Input: part model. Units: mm. Frame: model coordinates. Coordinates: 2 decimals unless noted, no trailing zeros. Write each loop counter-clockwise with the first axis right and the second up, starting at its lowest first coordinate (ties: lowest second). Pieces come first, ordered by that corner, then holes.
1) Section query C-C (z = 36). Output: boundary loops of the cut face in (x, y).
2) Line query: L1, parallel to Z at x = -1, y = 0.75; L2, parallel to X at y = 0.9, z = 45.5; L3, parallel to X at y = 0.7, z = -29.5. Output: solid intervals per line, ascending.
3) Section query B-B (x = -35). Output: boundary loops of the cut face in (y, z), then the cut area to 3 significant figures.
4) Section query A-A (y = 0.45). Output: boundary loops of the cut face in (x, z), then the cut area to 3 significant figures.
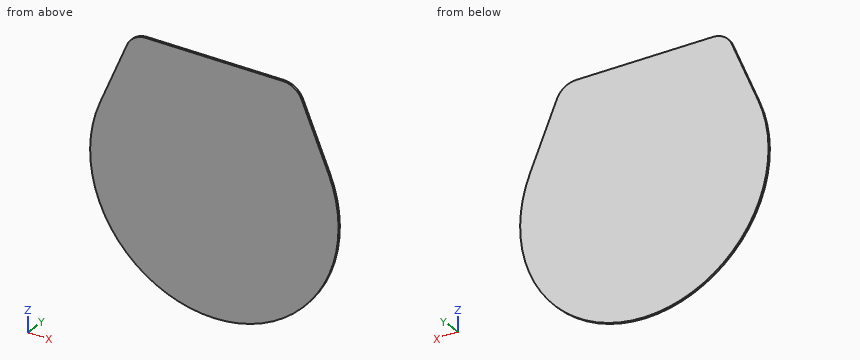
from build123d import *

# Parameters (mm, degrees)
SKETCH1_R           = 60.5
BOSS_EXTRUDE1_DEPTH = 1
BOSS_EXTRUDE2_START = -1
BOSS_EXTRUDE2_DEPTH = 1
FILLET1_R           = 10


with BuildPart() as part:
    # Sketch1 → Boss-Extrude1 (new body)
    with BuildSketch(Plane(origin=(0, 0, 0), x_dir=(1, 0, 0), z_dir=(0, 1, 0))):
        with Locations(Location((0, 0, 0), (0, 0, 270))):
            Circle(SKETCH1_R)
    extrude(amount=BOSS_EXTRUDE1_DEPTH)

    # Sketch7 → Boss-Extrude2 (add)
    with BuildSketch(Plane(origin=(0, 1, 0), x_dir=(1, 0, 0), z_dir=(0, 1, 0)).offset(BOSS_EXTRUDE2_START)):
        with BuildLine():
            Line((-55.577310907, -23.904236284), (-40, -60.5))
            Line((-40, -60.5), (2.22e-07, -60.5))
            ThreePointArc((2.22e-07, -60.5), (-33.271937819, -50.529478067), (-55.577310907, -23.904236284))
        make_face()
        with BuildLine():
            ThreePointArc((55.577310907, -23.904236284), (33.271938005, -50.529477945), (2.22e-07, -60.5))
            Line((2.22e-07, -60.5), (40, -60.5))
            Line((40, -60.5), (55.577310907, -23.904236284))
        make_face()
    extrude(amount=BOSS_EXTRUDE2_DEPTH)

    # Fillet1
    fillet1_edges = [part.edges().sort_by_distance(p)[0] for p in [
        (40, 0.5, 60.5),
        (-40, 0.5, 60.5),
    ]]
    fillet(fillet1_edges, radius=FILLET1_R)


solid = part.part
Answer:
1. outline: (-50.43, 0) - (50.43, 0) - (50.43, 1) - (-50.43, 1) - close
2. L1: z = -60.49 to 60.5
2. L2: x = -46.38 to 46.38
2. L3: x = -52.82 to 52.82
3. outline: (0, -49.35) - (1, -49.35) - (1, 60.37) - (0, 60.37) - close
3. area: 110 mm2
4. outline: (-55.58, 23.9) arc R60.5 ccw (long way) to (55.58, 23.9) - (42.59, 54.42) arc R10 ccw to (33.39, 60.5) - (-33.39, 60.5) arc R10 ccw to (-42.59, 54.42) - close
4. area: 12,000 mm2
